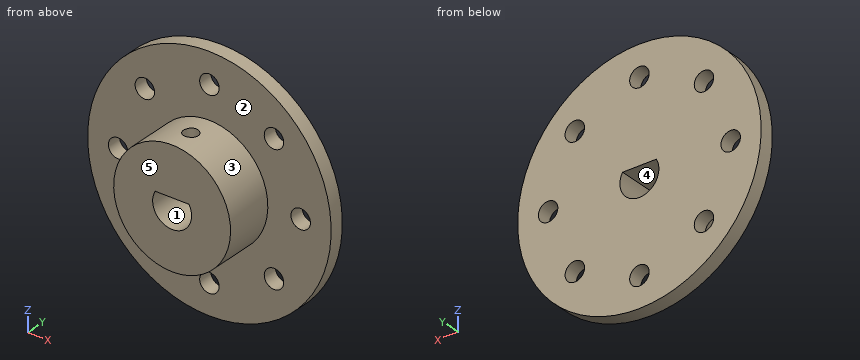
```python
from build123d import *

# Parameters (mm, degrees)
SKETCH_1_R          = 25
SKETCH_1_R_2        = 2
EXTRUDE_1_DEPTH     = 3
SKETCH_2_R          = 12
EXTRUDE_2_DEPTH     = 10
CUT_EXTRUDE_1_DEPTH = 38.669616404
SKETCH_4_R          = 1.5
CUT_EXTRUDE_2_DEPTH = 39.13135193


with BuildPart() as part:
    # 草图1 → 凸台-拉伸1 (new body)
    with BuildSketch(Plane(origin=(0, 0, 0), x_dir=(1, 0, 0), z_dir=(0, 1, 0))):
        with Locations(Location((0, 0, 0), (0, 0, 270))):
            Circle(SKETCH_1_R)
        with Locations(Location((-18.75, 0, 0), (0, 0, 270))):
            Circle(SKETCH_1_R_2, mode=Mode.SUBTRACT)
        with Locations(Location((0, -18.75, 0), (0, 0, 90))):
            Circle(SKETCH_1_R_2, mode=Mode.SUBTRACT)
        with Locations(Location((-13.258252147, -13.258252147, 0), (0, 0, 270))):
            Circle(SKETCH_1_R_2, mode=Mode.SUBTRACT)
        with Locations(Location((0, 18.75, 0), (0, 0, 270))):
            Circle(SKETCH_1_R_2, mode=Mode.SUBTRACT)
        with Locations(Location((-13.258252147, 13.258252147, 0), (0, 0, 90))):
            Circle(SKETCH_1_R_2, mode=Mode.SUBTRACT)
        with Locations(Location((13.258252147, 13.258252147, 0), (0, 0, 270))):
            Circle(SKETCH_1_R_2, mode=Mode.SUBTRACT)
        with Locations(Location((18.75, 0, 0), (0, 0, 90))):
            Circle(SKETCH_1_R_2, mode=Mode.SUBTRACT)
        with Locations(Location((13.258252147, -13.258252147, 0), (0, 0, 90))):
            Circle(SKETCH_1_R_2, mode=Mode.SUBTRACT)
    extrude(amount=EXTRUDE_1_DEPTH)

    # 草图2 → 凸台-拉伸2 (add)
    with BuildSketch(Plane.XZ):
        with Locations(Location((0, 0, 0), (0, 0, 270))):
            Circle(SKETCH_2_R)
    extrude(amount=EXTRUDE_2_DEPTH)

    # 草图3 → 切除-拉伸1 (cut, through all)
    with BuildSketch(Plane.XZ.offset(10)):
        with BuildLine():
            Line((-3.464101615, 2), (3.464101615, 2))
            ThreePointArc((3.464101615, 2), (0, -4), (-3.464101615, 2))
        make_face()
    extrude(amount=-CUT_EXTRUDE_1_DEPTH, mode=Mode.SUBTRACT)

    # 草图4 → 切除-拉伸2 (cut, through all)
    with BuildSketch(Plane(origin=(0, 0, 2), x_dir=(-1, 0, 0), z_dir=(0, 0, -1))):
        with Locations((0, -5)):
            Circle(SKETCH_4_R)
    extrude(amount=-CUT_EXTRUDE_2_DEPTH, mode=Mode.SUBTRACT)


solid = part.part
```
For this review, take the finished solid that the model builds, in its own axes (mm). Face numbers are marked on the shaded views. A direction names the side the tool comes from. Round coordinates to 2 decimals unless told otherwise and drop trailing zeros. Loops run counter-clockwise (first coordinate to the right, second up) from the corner with the lowest first, then second, coordinate; pieces in that order, holes last.
(1) We need section C-C (x = 14.5). Give the boundary of the cut face in (y, z).
Returned:
outline: (0, -20.37) - (3, -20.37) - (3, -14.83) - (0, -14.83) - close; (0, -11.69) - (3, -11.69) - (3, 11.69) - (0, 11.69) - close; (0, 14.83) - (3, 14.83) - (3, 20.37) - (0, 20.37) - close
(2) We need section D-D (z = 5). Give the boundary of the cut face in (x, y), plus the area to 3 significant figures.
Returned:
outline: (-24.49, 0) - (-10.91, 0) - (-10.91, -10) - (10.91, -10) - (10.91, 0) - (24.49, 0) - (24.49, 3) - (-24.49, 3) - close; hole circle Ø3 at (0, -5)
area: 358 mm2
(3) Tool access review of the marked faces 1 and 2: name each direction out of +Z, -Z, +X, -X, +Y, -Y from which nothing blocks a thin tool from reaching the whole face with its end or side.
Returned:
face 1: +Y, -Y
face 2: -Y
(4) Mouldability with a two-part tool opening along X and no side actions: class the marked faces 3, 4 and 5 as released by +X, released by -X, zero draft, split by the parting line, or undercut.
Returned:
face 3: split by the parting line
face 4: undercut
face 5: zero draft
(5) Wall thickness on line 1 along Z through (x, y) = (13.5, 1); line 2 along X through (y, z) = (1, -12.5); line 3 along X through (y, z) = (1.25, -12): over which ranges is each line inside the solid? List them lowest first.
Returned:
line 1: z = -21.04 to -15.24, -11.27 to 11.27, 15.24 to 21.04
line 2: x = -21.65 to -15.11, -11.41 to 11.41, 15.11 to 21.65
line 3: x = -21.93 to -14.81, -11.7 to 11.7, 14.81 to 21.93
(6) We need section A-A (z = 0). Give the boundary of the cut face in (x, y), plus the area to 3 significant figures.
Returned:
outline: (-25, 0) - (-20.75, 0) - (-20.75, 3) - (-25, 3) - close; (-16.75, 0) - (-12, 0) - (-12, -10) - (-4, -10) - (-4, 3) - (-16.75, 3) - close; (4, -10) - (12, -10) - (12, 0) - (16.75, 0) - (16.75, 3) - (4, 3) - close; (20.75, 0) - (25, 0) - (25, 3) - (20.75, 3) - close
area: 262 mm2
(7) We need section B-B (x = 0). Give the boundary of the cut face in (y, z), plus the area to 3 significant figures.
Returned:
outline: (-10, -12) - (0, -12) - (0, -16.75) - (3, -16.75) - (3, -4) - (-10, -4) - close; (-10, 2) - (-6.5, 2) - (-6.5, 12) - (-10, 12) - close; (-3.5, 2) - (3, 2) - (3, 16.75) - (0, 16.75) - (0, 12) - (-3.5, 12) - close; (0, -25) - (3, -25) - (3, -20.75) - (0, -20.75) - close; (0, 20.75) - (3, 20.75) - (3, 25) - (0, 25) - close
area: 258 mm2
(8) Clearance check with flat-ended pins moving along their axes: P1, Ø3, axis at x = 1, y = -8, coming from the -Z side; P2, Ø2.5, axis at x = 0, z = 18.75, coming from the +Y side; P3, Ø5, axis at x = -4.5, y = -6.5, coming from the +Z side; P4, Ø5, axis at x = 13.26, z = -13.26, coming from the +Y side. State where each tip first meets the part, or that it passes through.
Returned:
P1: stops at z = -12
P2: passes through
P3: stops at z = 11.83
P4: stops at y = 3
